Verification items for this drawing (mm, ordinates from the low corner). Coordinates: 2 decimals unless noted, no trailing zeros. Order: outer loops, then holes, each group sorted by start corner. A loop starts at its lowest first (then second) coordinate and runs counter-clockwise, first axis right, second up.
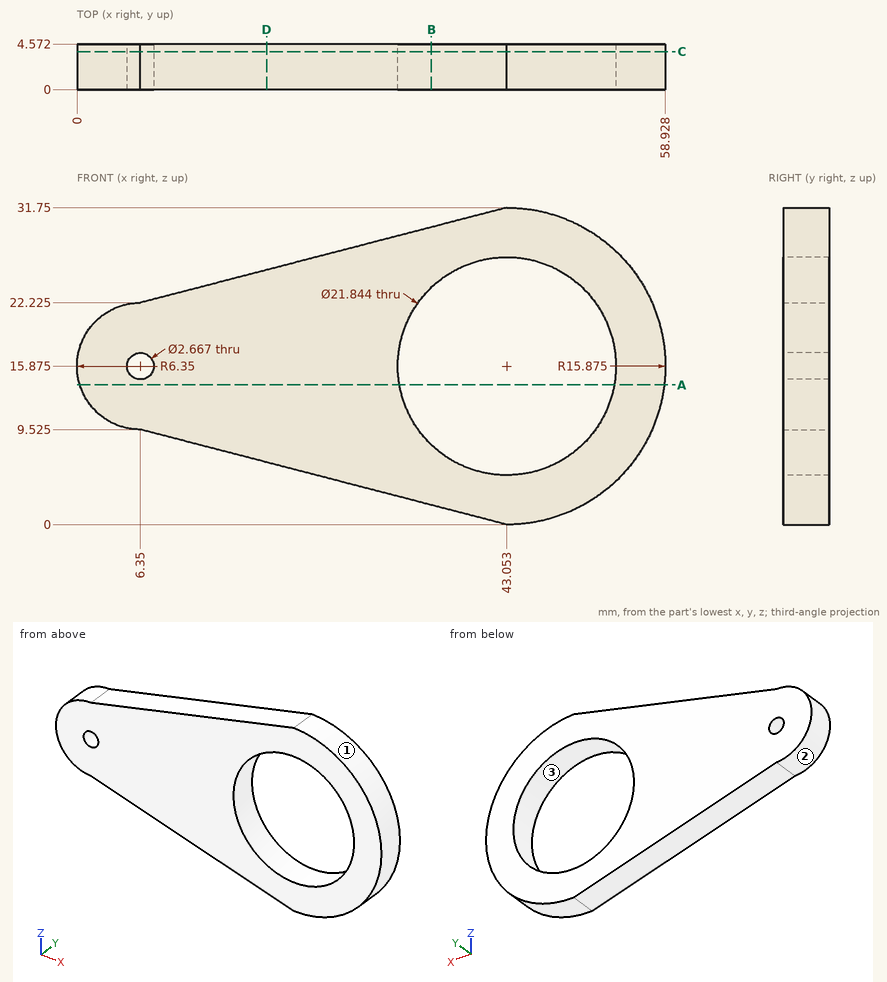
(1) Cross-section at A-A (z = 14). Enter the section's corners in (x, y), and give its area (3 significant figures).
Filled in:
outline: (0.28, 0) - (32.29, 0) - (32.29, 4.57) - (0.28, 4.57) - close; (53.81, 0) - (58.82, 0) - (58.82, 4.57) - (53.81, 4.57) - close
area: 169 mm2
(2) Release check for a two-part mould opening along X. For the marked faces 1, 2 and 3 record: +X half, -X half, draft (parallel to the pull), parting line (faces both ways), or undercut.
Filled in:
face 1: +X half
face 2: -X half
face 3: undercut
(3) Go/stop test with flat-tipped pins: P1, Ø2, axis at y = 0.5, z = 20, coming from the -X side; P2, Ø1.5, axis at x = 25.5, y = 2, coming from the -Z side. Record where each tip stops, or that it passes through.
Filled in:
P1: stops at x = 0.82
P2: stops at z = 4.36
(4) Thickness scan on probe 1 along X at (y, z) = (2.6, 16.5); probe 2 along X at (y, z) = (4.2, 15); probe 3 along Z at (x, y) = (7, 3.35). Record the ranges inside material, lowest first.
Filled in:
probe 1: x = 0.03 to 5.17, 7.53 to 32.15, 53.96 to 58.92
probe 2: x = 0.06 to 5.34, 7.36 to 32.17, 53.94 to 58.9
probe 3: z = 9.36 to 14.71, 17.04 to 22.39
(5) Cross-section at B-B (x = 35.5). Enter the section's corners in (y, z).
Filled in:
outline: (0, 1.96) - (4.57, 1.96) - (4.57, 7.99) - (0, 7.99) - close; (0, 23.76) - (4.57, 23.76) - (4.57, 29.79) - (0, 29.79) - close
(6) Cross-section at C-C (y = 3.8). Count the separate pieces of the cut face and the enclosed holes in it, and give its area (3 significant figures).
Filled in:
separate pieces: 1
enclosed holes: 2
area: 895 mm2
(7) Cross-section at D-D (x = 19). Enter the section's corners in (y, z).
Filled in:
outline: (0, 6.24) - (4.57, 6.24) - (4.57, 25.51) - (0, 25.51) - close
